For this review, take the finished solid that the model builds, in its own axes (mm). A direction names the side the tool comes from. Give positions to 0.01 mm unless a question says otherwise; leave off trailing zeros. Order: outer loops, then holes, each group sorted by start corner. A loop starts at its lowest first (then second) coordinate and runs counter-clockwise, first axis right, second up. Notation, with made-up numbers: M -32,42 L -1,42 A33 ccw -1,79 Z; hole C 50,-16 d6. An arc over 180 degrees is marked long. Answer as CSV lines item,"result". Start each with the question number.
1. We need section B-B, the plane z = 28. Give the boundary of the cut face in (x, y).
2. For line 1 along Z through (x, y) = (7, 72); line 2 along X through (y, z) = (76, 19), list the stretches that pass through material, from the lowest coordinate up.
3. Machinability: for faces 5 (the flat face through (19, 49, 2)), 6 (the flat face through (0, 49, 25)), which of the approach directions +Z, -Z, +X, -X, +Y, -Y give a long, thin tool a straight path to every point of the face, cutting with its end or side? Answer none if there is none.
4. We need section C-C, the plane x = 8. Give the boundary of the cut face in (y, z), and give its area (3 significant figures).
5. Mouldability with a two-part tool opening along Z and no side actions: class faces 1 (the flat face through (18, 49, 48)), 2 (the flat face through (1, 0, 27)), 3 (the flat face through (18, 51, 50)), 4 (the flat face through (2, 48, 25)) as pulls with the +Z half, pulls with the -Z half, needs draft (parallel to the pull), parting line crosses it, or undercut.
6. We need section A-A, the plane y = 40. Give the boundary of the cut face in (x, z), and give its area (3 significant figures).
Autodesk Inventor part; units mm, degrees
ref_plane "YZ Plane" through (0, 0, 0) normal (1, 0, 0) x (0, 1, 0)
ref_plane "XZ Plane" through (0, 0, 0) normal (0, 1, 0) x (-1, 0, 0)
ref_plane "XY Plane" through (0, 0, 0) normal (0, 0, 1) x (1, 0, 0)
sketch "Sketch1" plane through (0, 0, 0) normal (0, 0, 1) x (1, 0, 0)
  line L0 (0, 0) -> (37, 0)
  line L1 (37, 0) -> (37, 100)
  line L2 (0, 96.7629) -> (0, 0)
  line L3 (37, 100) -> (0, 96.7629)
  line L4 (37, 100) -> (74.1413, 100) construction
  dimension "d0" = 37
  dimension "d1" = 100
  dimension "d2" = 175
extrude "Extrusion1" add sketch "Sketch1" along normal blind 50
sketch "Sketch2" plane through (0, 0, 0) normal (0, -1, 0) x (1, 0, 0)
  line L0 (35, 48) -> (35, 2)
  line L1 (37, 0) -> (0, 0)
  line L2 (35, 2) -> (2, 2)
  line L3 (2, 2) -> (2, 48)
  line L4 (2, 48) -> (35, 48)
  dimension "d5" = 46
  dimension "d6" = 33
extrude "Extrusion2" cut sketch "Sketch2" against normal blind 100
properties part number "Housing of the motor"
Result set:
1,outline,"M 0,0 L 2,0 L 2,96.94 L 0,96.76 Z; M 35,0 L 37,0 L 37,100 L 35,99.83 Z"
2,line 1,"0 to 2, 48 to 50"
2,line 2,"0 to 2, 35 to 37"
3,face 5,"+Y, -Y"
3,face 6,"+Z, -Z, -X, +Y, -Y"
4,outline,"M 0,0 L 97.46,0 L 97.46,2 L 0,2 Z; M 0,48 L 97.46,48 L 97.46,50 L 0,50 Z"
4,area,"390 mm2"
5,face 1,"undercut"
5,face 2,"needs draft"
5,face 3,"pulls with the +Z half"
5,face 4,"undercut"
6,outline,"M 0,0 L 37,0 L 37,50 L 0,50 Z; hole M 2,2 L 35,2 L 35,48 L 2,48 Z"
6,area,"332 mm2"
